from build123d import *

# Parameters (mm, degrees)
PAD_DEPTH        = 10
HOLE_D           = 6.6
HOLE_DEPTH       = 25
HOLE_CBORE_D     = 11
HOLE_CBORE_DEPTH = 6.4
FILLET_R         = 2


with BuildPart() as part:
    # Sketch → Pad (new body)
    with BuildSketch(Plane.XY):
        with BuildLine():
            Line((-34.5, 25), (34.5, 25))
            ThreePointArc((37.5, 22), (36.62132, 24.12132), (34.5, 25))
            Line((37.5, 22), (37.5, -22))
            ThreePointArc((34.5, -25), (36.62132, -24.12132), (37.5, -22))
            Line((34.5, -25), (-33.596236, -25))
            ThreePointArc((-37.5, -21.096236), (-36.356614, -23.856614), (-33.596236, -25))
            Line((-37.5, -21.096236), (-37.5, 22))
            ThreePointArc((-34.5, 25), (-36.62132, 24.12132), (-37.5, 22))
        make_face()
        with BuildLine():
            ThreePointArc((-22, 17), (-25, 20), (-28, 17))
            Line((-28, 17), (-28, -17))
            ThreePointArc((-28, -17), (-25, -20), (-22, -17))
            Line((-22, -17), (-22, 17))
        make_face(mode=Mode.SUBTRACT)
        with BuildLine():
            ThreePointArc((28, 17), (25, 20), (22, 17))
            Line((22, 17), (22, -17))
            ThreePointArc((22, -17), (25, -20), (28, -17))
            Line((28, -17), (28, 17))
        make_face(mode=Mode.SUBTRACT)
    extrude(amount=PAD_DEPTH)

    # Hole
    with Locations(Plane(origin=(0, 0, 0), x_dir=(1, 0, 0), z_dir=(0, 0, -1))):
        with Locations((0, 0), (0, 12.5), (0, -12.5)):
            CounterBoreHole(HOLE_D / 2, HOLE_CBORE_D / 2, HOLE_CBORE_DEPTH, depth=HOLE_DEPTH)

    # Fillet
    fillet_edges = [part.edges().sort_by_distance(p)[0] for p in [
        (0.451882, -25, 10),
    ]]
    fillet(fillet_edges, radius=FILLET_R)


solid = part.part
Source: CAD feature listing. Evaluate the final solid. Frame: model axes, mm. A direction names the side the tool comes from. Round coordinates to 2 decimals unless told otherwise and drop trailing zeros. Loops run counter-clockwise (first coordinate to the right, second up) from the corner with the lowest first, then second, coordinate; pieces in that order, holes last. Notation, with made-up numbers: (11.25, -9.5) - (46.25, -9.5) arc R14 ccw to (46.25, -2.5) - close; hole circle Ø8 at (33.25, 31.5). An arc over 180 degrees is marked (long way). Write item = value, one per line. Start each with the question number.
(1) Section query D-D, the plane x = 24. Output: boundary loops of the cut face in (y, z), plus the area to 3 significant figures.
(2) Pin query (flat end, axial travel): pin 1 (3.5 mm diameter, centred on x = 1, y = -1.5, fed in from -Z); pin 2 (6.5 mm diameter, centred on x = 0, y = 12.5, fed in from -Z). Return the tip coordinate at first contact, or that it passes through.
(3) Section query A-A, the plane y = -12.5. Output: boundary loops of the cut face in (x, z), plus the area to 3 significant figures.
(4) Section query B-B, the plane x = -25. Output: boundary loops of the cut face in (y, z).
(5) Section query C-C, the plane z = 4.25. Output: boundary loops of the cut face in (x, y), plus the area to 3 significant figures.
(6) Pull-direction query (X, two-part tool) for faces 1 (the face through (2.43, -2.23, 8.23)), 2 (the face through (0.48, 24.4, 9.43)), 3 (the face through (-28, 0, 5)), 4 (the face through (36.64, 24.1, 3.94)); classes: +X half, -X half, draft (parallel to the pull), parting line (faces both ways), or undercut.
(7) Ray query, line 1 along X through (y, z) = (-6, 4); line 2 along Y through (x, z) = (0, 4.75); line 3 along X through (y, z) = (8, 9.5). Return the intervals inside material, ascending. Write a range as from..to.
(8) Set-up query: faces 5 (the face through (-1.19, 17.87, 3.16)), 6 (the face through (1, -25, 4)), 7 (the face through (-25, 20, 5)). Return all of +Z, -Z, +X, -X, +Y, -Y with unobstructed straight access to the full face (end or side cutting, diameter ignored); none if empty.
Conclusion:
q1.outline = (-25, 0) - (-19.83, 0) - (-19.83, 10) - (-23, 10) arc R2 ccw to (-25, 8) - close; (19.83, 0) - (25, 0) - (25, 8) arc R2 ccw to (23, 10) - (19.83, 10) - close
q1.area = 102 mm2
q2.pin_1 = 6.4
q2.pin_2 = through
q3.outline = (-37.5, 0) - (-28, 0) - (-28, 10) - (-35.5, 10) arc R2 ccw to (-37.5, 8) - close; (-22, 0) - (-5.5, 0) - (-5.5, 6.4) - (-3.3, 6.4) - (-3.3, 10) - (-22, 10) - close; (3.3, 6.4) - (5.5, 6.4) - (5.5, 0) - (22, 0) - (22, 10) - (3.3, 10) - close; (28, 0) - (37.5, 0) - (37.5, 8) arc R2 ccw to (35.5, 10) - (28, 10) - close
q3.area = 534 mm2
q4.outline = (-25, 0) - (-20, 0) - (-20, 10) - (-23, 10) arc R2 ccw to (-25, 8) - close; (20, 0) - (25, 0) - (25, 8) arc R2 ccw to (23, 10) - (20, 10) - close
q5.outline = (-37.5, -21.1) arc R3.9 ccw to (-33.6, -25) - (34.5, -25) arc R3 ccw to (37.5, -22) - (37.5, 22) arc R3 ccw to (34.5, 25) - (-34.5, 25) arc R3 ccw to (-37.5, 22) - close; hole (-28, -17) arc R3 ccw to (-22, -17) - (-22, 17) arc R3 ccw to (-28, 17) - close; hole circle Ø11 at (0, -12.5); hole circle Ø11 at (0, 0); hole circle Ø11 at (0, 12.5); hole (22, -17) arc R3 ccw to (28, -17) - (28, 17) arc R3 ccw to (22, 17) - close
q5.area = 2,990 mm2
q6.face_1 = undercut
q6.face_2 = draft
q6.face_3 = undercut
q6.face_4 = +X half
q7.line_1 = -37.5..-28, -22..22, 28..37.5
q7.line_2 = -25..-18, -7..-5.5, 5.5..7, 18..25
q7.line_3 = -36.82..-28, -22..22, 28..36.82
q8.face_5 = -Z
q8.face_6 = +Z, -Z, +X, -X, -Y
q8.face_7 = +Z, -Z
